Autodesk Inventor part; units mm, degrees
ref_plane "YZ Plane" through (0, 0, 0) normal (1, 0, 0) x (0, 1, 0)
ref_plane "XZ Plane" through (0, 0, 0) normal (0, 1, 0) x (-1, 0, 0)
ref_plane "XY Plane" through (0, 0, 0) normal (0, 0, 1) x (1, 0, 0)
sketch "Sketch3" plane through (0, 0, 0) normal (0, 0, 1) x (1, 0, 0)
  circle A0 centre (0, 0) radius 9.525
  circle A1 centre (0, 0) radius 3
  circle A2 centre (6.2, 0) radius 1.5
  circle A3 centre (3.1, 5.3694) radius 1.5
  circle A4 centre (-3.1, 5.3694) radius 1.5
  circle A5 centre (-6.2, 0) radius 1.5
  circle A6 centre (-3.1, -5.3694) radius 1.5
  circle A7 centre (3.1, -5.3694) radius 1.5
  dimension "d0" = 19.05
  dimension "d1" = 6
  dimension "d4" = 3
  dimension "d5" = 6.2
  dimension "d12" = 360
extrude "Extrusion1" add sketch "Sketch3" along normal blind 9.525 contours A0 | A2 | A3 | A4 | A5 | A6 | A7
sketch "Sketch7" plane through (0, 0, 0) normal (0, 1, 0) x (-1, 0, 0)
  circle A0 centre (0, 4.7625) radius 2.5
  line L0 (-9.525, 0) -> (-9.525, 9.525)
  point P0 (0, 0)
  point P1 (-9.525, 4.7625)
  dimension "d42" = 5
extrude "Extrusion5" cut sketch "Sketch7" against normal through all
sketch "Sketch8" plane through (0, 0, 0) normal (0, 0, -1) x (-1, 0, 0)
  circle A0 centre (0, 6.35) radius 2
  circle A1 centre (-5.5026, -3.1692) radius 2
  circle A2 centre (5.4925, -3.1867) radius 2
  circle A3 centre (0.0202, 6.35) radius 2
  point P0 (0, 0)
  dimension "d45" = 4
  dimension "d46" = 6.35
  dimension "d49" = 359.817
extrude "Extrusion6" cut sketch "Sketch8" against normal through all contours A0 A3 | A3 A0 | A1 | A2 picked at (-0.6435, 6.35) picked at (-1.9787, 6.4301)
properties part number "6mm Mounting Hub, thin" material "Aluminum 6061"
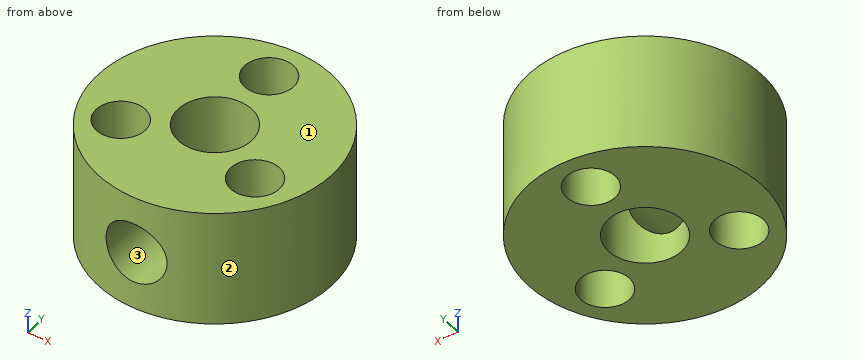
Can you work these out from the model? Positions are in its coordinate system, mm. Face numbers are marked on the shaded views. Coordinates: 2 decimals unless noted, no trailing zeros. Loops run counter-clockwise (first coordinate to the right, second up) from the corner with the lowest first, then second, coordinate; pieces in that order, holes last. Notation, with made-up numbers: (31.25, 40.25) - (83.25, 40.25) arc R17 ccw to (83.25, 64.25) - close; hole circle Ø5 at (30, 25). An arc over 180 degrees is marked (long way). Use a Markdown table: item, result.
Item 1: If I drill on probe 1 along Y at (x, z) = (-0.75, 7.5); probe 2 along Y at (x, z) = (0, 3.75) (3 decimals); probe 3 along Y at (x, z) = (-4.5, 8.75), over which ranges is the centre line in solid material (lowest first)? Write a range as from..to.
Numbers:
| item | result |
|---|---|
| probe 1 | y = -9.5..-2.9, 2.9..4.5, 8.2..9.5 |
| probe 2 | y = 3..4.35, 8.35..9.525 |
| probe 3 | y = -8.39..-4.92, -1.45..8.39 |
Item 2: I want a section at B-B on x = 0. Give the number of separate pieces and of enclosed holes in the cut face, and give its area (3 significant figures).
Numbers:
| item | result |
|---|---|
| separate pieces | 4 |
| enclosed holes | 0 |
| area | 53.6 mm2 |
Item 3: I want a section at D-D on x = 4.5. Please give me the cut outline in (y, z) (3 decimals).
Numbers:
| item | result |
|---|---|
| outline | (-8.395, 0) - (-4.9, 0) - (-4.9, 9.525) - (-8.395, 9.525) - close; (-1.439, 0) - (8.395, 0) - (8.395, 9.525) - (-1.439, 9.525) - close |
Item 4: I want a section at A-A on y = 0. Please give me the cut outline in (x, z) (3 decimals), and give its area (3 significant figures).
Numbers:
| item | result |
|---|---|
| outline | (-9.525, 0) - (-3, 0) - (-3, 9.525) - (-9.525, 9.525) - close; (3, 0) - (9.525, 0) - (9.525, 9.525) - (3, 9.525) - close |
| area | 124 mm2 |
Item 5: We'd pull the mould along X, two halves only. Please class the marked faces 1, 2 and 3: released by +X, released by -X, zero draft, split by the parting line, or undercut.
Numbers:
| item | result |
|---|---|
| face 1 | zero draft |
| face 2 | split by the parting line |
| face 3 | undercut |
Item 6: Will these pins go through, and if not, where does the flat tip stop? pin 1 (1 mm diameter, centred on x = -6.5, z = 2.5, fed in from +Y); pin 2 (5 mm diameter, centred on x = 0, y = 0, fed in from +Z); pin 3 (1.5 mm diameter, centred on y = -1.5, z = 8, fed in from -X); pin 4 (1 mm diameter, centred on y = -4, z = 1.5, fed in from +X).
Numbers:
| item | result |
|---|---|
| pin 1 | stops at y = 7.4 |
| pin 2 | passes through |
| pin 3 | stops at x = -9.5 |
| pin 4 | stops at x = 8.86 |
Item 7: I want a section at C-C on y = -4.5. Please give me the cut outline in (x, z) (1 decimal).
Numbers:
| item | result |
|---|---|
| outline | (-8.4, 0) - (-7, 0) - (-7, 9.5) - (-8.4, 9.5) - close; (-4, 0) - (4, 0) - (4, 9.5) - (-4, 9.5) - close; (7, 0) - (8.4, 0) - (8.4, 9.5) - (7, 9.5) - close; hole circle Ø5 at (0, 4.8) |
